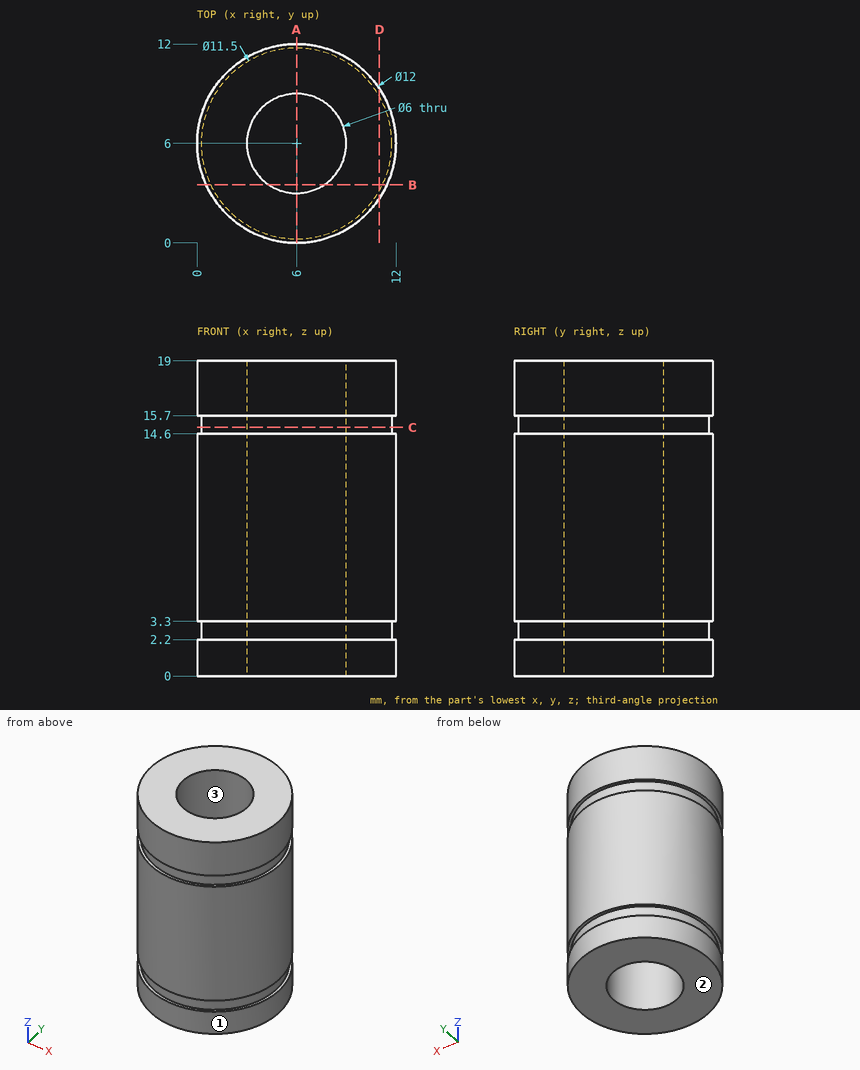
Drawing for the job (mm, zero at the part's lowest x, y, z). Round coordinates to 2 decimals unless told otherwise and drop trailing zeros. Order: outer loops, then holes, each group sorted by start corner. A loop starts at its lowest first (then second) coordinate and runs counter-clockwise, first axis right, second up.
Item 1: Mould opens along X. For the marked faces 1, 2 and 3 say: pulls with the +X half, pulls with the -X half, needs draft (parallel to the pull), parting line crosses it, or undercut.
Item 2: Saw through at C-C on z = 15. Write the cut outline in (x, y), then the cut area to 3 significant figures.
Item 3: Saw through at D-D on x = 11. Write the cut outline in (y, z).
Item 4: Pin check, flat tips, straight feed: pin 1 (1.5 mm diameter, centred on y = 3.5, z = 16.5, fed in from +X); pin 2 (5 mm diameter, centred on x = 9, z = 11.5, fed in from -Y); pin 3 (5 mm diameter, centred on y = 2, z = 2.5, fed in from +X). Stop position of each tip, or through.
Item 5: Saw through at A-A on x = 6. Write the cut outline in (y, z), then the cut area to 3 significant figures.
Item 6: Probe line 1 along Z through (x, y) = (11, 3); line 2 along Y through (x, z) = (6, 13); line 3 along Y through (x, z) = (8.5, 15.25). List the from-to ranges inside material, lowest first.
Item 7: Saw through at B-B on y = 3.5. Write the cut outline in (x, z), then the cut area to 3 significant figures.
Reported:
1. face 1: parting line crosses it
1. face 2: needs draft
1. face 3: undercut
2. outline: circle Ø11.5 at (6, 6); hole circle Ø6 at (6, 6)
2. area: 75.6 mm2
3. outline: (2.68, 0) - (9.32, 0) - (9.32, 2.2) - (8.84, 2.2) - (8.84, 3.3) - (9.32, 3.3) - (9.32, 14.6) - (8.84, 14.6) - (8.84, 15.7) - (9.32, 15.7) - (9.32, 19) - (2.68, 19) - (2.68, 15.7) - (3.16, 15.7) - (3.16, 14.6) - (2.68, 14.6) - (2.68, 3.3) - (3.16, 3.3) - (3.16, 2.2) - (2.68, 2.2) - close
4. pin 1: stops at x = 11.74
4. pin 2: stops at y = 0.02
4. pin 3: stops at x = 11.8
5. outline: (0, 0) - (3, 0) - (3, 19) - (0, 19) - (0, 15.7) - (0.25, 15.7) - (0.25, 14.6) - (0, 14.6) - (0, 3.3) - (0.25, 3.3) - (0.25, 2.2) - (0, 2.2) - close; (9, 0) - (12, 0) - (12, 2.2) - (11.75, 2.2) - (11.75, 3.3) - (12, 3.3) - (12, 14.6) - (11.75, 14.6) - (11.75, 15.7) - (12, 15.7) - (12, 19) - (9, 19) - close
5. area: 113 mm2
6. line 1: z = 0 to 2.2, 3.3 to 14.6, 15.7 to 19
6. line 2: y = 0 to 3, 9 to 12
6. line 3: y = 0.82 to 4.34, 7.66 to 11.18
7. outline: (0.55, 0) - (4.34, 0) - (4.34, 19) - (0.55, 19) - (0.55, 15.7) - (0.82, 15.7) - (0.82, 14.6) - (0.55, 14.6) - (0.55, 3.3) - (0.82, 3.3) - (0.82, 2.2) - (0.55, 2.2) - close; (7.66, 0) - (11.45, 0) - (11.45, 2.2) - (11.18, 2.2) - (11.18, 3.3) - (11.45, 3.3) - (11.45, 14.6) - (11.18, 14.6) - (11.18, 15.7) - (11.45, 15.7) - (11.45, 19) - (7.66, 19) - close
7. area: 143 mm2
